Check sheet for the modelled part. Datum: model origin and axes. Units: mm. Coordinates: 2 decimals unless noted, no trailing zeros. Order: outer loops, then holes, each group sorted by start corner. A loop starts at its lowest first (then second) coordinate and runs counter-clockwise, first axis right, second up.
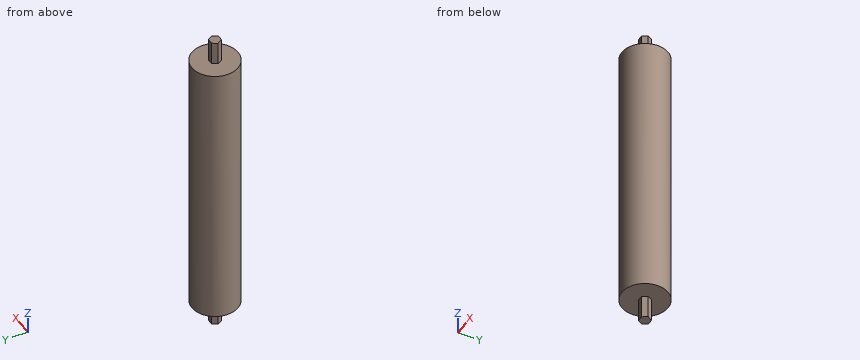
from build123d import *

# Parameters (mm, degrees)
SKETCH1_R           = 25.4
BOSS_EXTRUDE1_DEPTH = 300
BOSS_EXTRUDE2_DEPTH = 25.4
BOSS_EXTRUDE3_DEPTH = 25.4


with BuildPart() as part:
    # Sketch1 → Boss-Extrude1 (new body)
    with BuildSketch(Plane.XY):
        Circle(SKETCH1_R)
    extrude(amount=BOSS_EXTRUDE1_DEPTH)

    # Sketch2 → Boss-Extrude2 (add)
    with BuildSketch(Plane.XY.offset(300)):
        Polygon((6.408587988, 0), (3.204293994, 5.55), (-3.204293994, 5.55), (-6.408587988, 0), (-3.204293994, -5.55), (3.204293994, -5.55), align=None)
    extrude(amount=BOSS_EXTRUDE2_DEPTH)

    # Sketch3 → Boss-Extrude3 (add)
    with BuildSketch(Plane(origin=(0, 0, 0), x_dir=(-1, 0, 0), z_dir=(0, 0, -1))):
        Polygon((6.408587988, 0), (3.204293994, 5.55), (-3.204293994, 5.55), (-6.408587988, 0), (-3.204293994, -5.55), (3.204293994, -5.55), align=None)
    extrude(amount=BOSS_EXTRUDE3_DEPTH)


solid = part.part
(1) Cross-section at A-A (x = 0). Enter the section's corners in (y, z).
Filled in:
outline: (-25.4, 0) - (-5.55, 0) - (-5.55, -25.4) - (5.55, -25.4) - (5.55, 0) - (25.4, 0) - (25.4, 300) - (5.55, 300) - (5.55, 325.4) - (-5.55, 325.4) - (-5.55, 300) - (-25.4, 300) - close
(2) Go/stop test with flat-tipped pins: P1, Ø10, axis at x = -14, z = 209, coming from the -Y side; P2, Ø3, axis at x = -1.5, z = 318, coming from the -Y side; P3, Ø2, axis at x = -11, z = 41, coming from the -Y side. Record where each tip stops, or that it passes through.
Filled in:
P1: stops at y = -23.75
P2: stops at y = -5.55
P3: stops at y = -23.35
(3) Cross-section at D-D (y = -9.5). Enter the section's corners in (x, z).
Filled in:
outline: (-23.56, 0) - (23.56, 0) - (23.56, 300) - (-23.56, 300) - close
(4) Cross-section at C-C (y = 13). Enter the section's corners in (x, z), and give its area (3 significant figures).
Filled in:
outline: (-21.82, 0) - (21.82, 0) - (21.82, 300) - (-21.82, 300) - close
area: 13,100 mm2
(5) Thickness scan on probe 1 along Z at (x, y) = (-10.5, 9.5); probe 2 along Y at (x, z) = (-1, 184); probe 3 along X at (y, z) = (-2, 32). Record the ranges inside material, lowest first.
Filled in:
probe 1: z = 0 to 300
probe 2: y = -25.38 to 25.38
probe 3: x = -25.32 to 25.32
(6) Cross-section at B-B (z = 231.5). Enter the section's corners in (x, y).
Filled in:
outline: circle Ø50.8 at (0, 0)
